Here's how the part is built. I have some questions about the finished solid (model axes, mm). A direction names the side the tool comes from. Coordinates: 2 decimals unless noted, no trailing zeros. Write each loop counter-clockwise with the first axis right and the second up, starting at its lowest first coordinate (ties: lowest second). Pieces come first, ordered by that corner, then holes. Notation, with made-up numbers: M 10,45.5 L 58,45.5 A15 ccw 58,64.5 Z; hole C 45.5,22 d7. An arc over 180 degrees is marked long. Write each question's results on one line, items separated by ' | '. Start each with the question number.
from build123d import *

# Parameters (mm, degrees)
SKETCH_1_W          = 90
SKETCH_1_H          = 50
EXTRUDE_1_DEPTH     = 35
SKETCH_2_W          = 86
SKETCH_2_H          = 46
CUT_EXTRUDE_1_DEPTH = 32
SKETCH_3_R          = 6
CUT_EXTRUDE_2_DEPTH = 2
SKETCH_4_R          = 13
SKETCH_4_R_2        = 6
EXTRUDE_2_DEPTH     = 11
SKETCH_5_R          = 13
SKETCH_5_R_2        = 6
EXTRUDE_4_DEPTH     = 12
SKETCH_6_W          = 65
SKETCH_6_H          = 5
CUT_EXTRUDE_3_DEPTH = 51
SKETCH_7_W          = 3
SKETCH_7_H          = 15
CUT_EXTRUDE_4_DEPTH = 30
EXTRUDE_5_DEPTH     = 110
SKETCH_9_W          = 50
SKETCH_9_H          = 40
SKETCH_9_R          = 16
EXTRUDE_6_DEPTH     = 2
SKETCH_10_W         = 2
SKETCH_10_H         = 46
EXTRUDE_7_DEPTH     = 38
SKETCH_11_R         = 15
CUT_EXTRUDE_5_DEPTH = 10


with BuildPart() as part:
    # 草圖1 → 填料-伸長1 (new body)
    with BuildSketch(Plane(origin=(0, 0, 0), x_dir=(1, 0, 0), z_dir=(0, 1, 0))):
        Rectangle(SKETCH_1_W, SKETCH_1_H)
    extrude(amount=EXTRUDE_1_DEPTH)

    # 草圖2 → 除料-伸長1 (cut)
    with BuildSketch(Plane(origin=(0, 35, 0), x_dir=(1, 0, 0), z_dir=(0, 1, 0))):
        Rectangle(SKETCH_2_W, SKETCH_2_H)
    extrude(amount=-CUT_EXTRUDE_1_DEPTH, mode=Mode.SUBTRACT)

    # 草圖3 → 除料-伸長2 (cut)
    with BuildSketch(Plane.ZY.offset(45)):
        with Locations((0, 20)):
            Circle(SKETCH_3_R)
    extrude(amount=-CUT_EXTRUDE_2_DEPTH, mode=Mode.SUBTRACT)

    # 草圖4 → 填料-伸長2 (add)
    with BuildSketch(Plane.ZY.offset(-43)):
        with Locations((0, 20)):
            Circle(SKETCH_4_R)
        with Locations((0, 20)):
            Circle(SKETCH_4_R_2, mode=Mode.SUBTRACT)
    extrude(amount=EXTRUDE_2_DEPTH)

    # 草圖5 → 填料-伸長4 (add)
    with BuildSketch(Plane(origin=(-43, 0, 0), x_dir=(0, 0, -1), z_dir=(1, 0, 0))):
        with Locations((0, 20)):
            Circle(SKETCH_5_R)
        with Locations((0, 20)):
            Circle(SKETCH_5_R_2, mode=Mode.SUBTRACT)
    extrude(amount=-EXTRUDE_4_DEPTH)

    # 草圖6 → 除料-伸長3 (cut, through all)
    with BuildSketch(Plane(origin=(0, 0, -25), x_dir=(-1, 0, 0), z_dir=(0, 0, -1))):
        with Locations((10.5, 20)):
            Rectangle(SKETCH_6_W, SKETCH_6_H)
    extrude(amount=-CUT_EXTRUDE_3_DEPTH, mode=Mode.SUBTRACT)

    # 草圖7 → 除料-伸長4 (cut)
    with BuildSketch(Plane(origin=(45, 0, 0), x_dir=(0, 0, -1), z_dir=(1, 0, 0))):
        with Locations((-16.5, 20)):
            Rectangle(SKETCH_7_W, SKETCH_7_H)
        with Locations((16.5, 20)):
            Rectangle(SKETCH_7_W, SKETCH_7_H)
    extrude(amount=-CUT_EXTRUDE_4_DEPTH, mode=Mode.SUBTRACT)

    # 草圖8 → 填料-伸長5 (add)
    with BuildSketch(Plane.ZY.offset(45)):
        Polygon((-25, 35), (-23, 35), (-23, 2), (23, 2), (23, 35), (25, 35), (25, 0), (23, 0), (-23, 0), (-25, 0), align=None)
    extrude(amount=EXTRUDE_5_DEPTH)

    # 草圖9 → 填料-伸長6 (add)
    with BuildSketch(Plane.ZY.offset(155)):
        with Locations((0, 20)):
            Rectangle(SKETCH_9_W, SKETCH_9_H)
        with Locations((0, 20)):
            Circle(SKETCH_9_R, mode=Mode.SUBTRACT)
    extrude(amount=EXTRUDE_6_DEPTH)

    # 草圖10 → 填料-伸長7 (add)
    with BuildSketch(Plane(origin=(0, 2, 0), x_dir=(1, 0, 0), z_dir=(0, 1, 0))):
        with Locations((-104, 0)):
            Rectangle(SKETCH_10_W, SKETCH_10_H)
    extrude(amount=EXTRUDE_7_DEPTH)

    # 草圖11 → 除料-伸長5 (cut)
    with BuildSketch(Plane.ZY.offset(105)):
        with Locations((0, 20)):
            Circle(SKETCH_11_R)
    extrude(amount=-CUT_EXTRUDE_5_DEPTH, mode=Mode.SUBTRACT)


solid = part.part
1) I want a section at B-B, the plane x = -112. Write out the boundary of the cut face in (y, z), then the cut area to 3 significant figures.
2) Please list where these lines run through material, in increasing order: line 1 (X direction, y = 26, z = -19); line 2 (X direction, y = 2.5, z = 17.5); line 3 (X direction, y = 7.5, z = -7.5). Write a range as [from, to].
3) We'd pull the mould along X, two halves only. Please class faces 1 (the flat face through (-130, 2, 0)), 2 (the flat face through (-55, 35, 24)), 3 (the flat face through (-155, 34, -11)), 4 (the flat face through (45, 17, 0)): pulls with the +X half, pulls with the -X half, needs draft (parallel to the pull), parting line crosses it, or undercut.
4) For pin 1 Ø0.6 at (x, z) = (-24, 24) entering from +Y; pin 2 Ø5 at (y, z) = (12, -3.5) entering from -X; pin 3 Ø3.5 at (y, z) = (17.5, 3) entering from -X, each with a flat end and sliding along its axis, tell me the tip position at first contact or that it passes through.
5) I want a section at A-A, the plane z = -9.5. Give the number of separate pieces and of enclosed holes in the cut face, then the cut area to 3 significant figures.
6) For faces 5 (the flat face through (-74, 2, 0)), 6 (the flat face through (-130, 18, 23)), 7 (the cylindrical face through (-155.99, 4.38, -3.47)), which set-ups out of +Z, -Z, +X, -X, +Y, -Y let a thin tool reach every point of the face, with its end or its side?
Output:
1) outline: M 0,-25 L 35,-25 L 35,-23 L 2,-23 L 2,23 L 35,23 L 35,25 L 0,25 Z | area: 232 mm2
2) line 1: x = [-157, -155], [-105, -103], [-45, -43], [43, 45] | line 2: x = [-157, -155], [-105, -103], [-45, 45] | line 3: x = [-45, -43], [43, 45]
3) face 1: undercut | face 2: needs draft | face 3: undercut | face 4: pulls with the +X half
4) pin 1: stops at y = 35 | pin 2: stops at x = -55 | pin 3: stops at x = 43
5) separate pieces: 3 | enclosed holes: 0 | area: 1,050 mm2
6) face 5: none | face 6: +Y | face 7: -X
